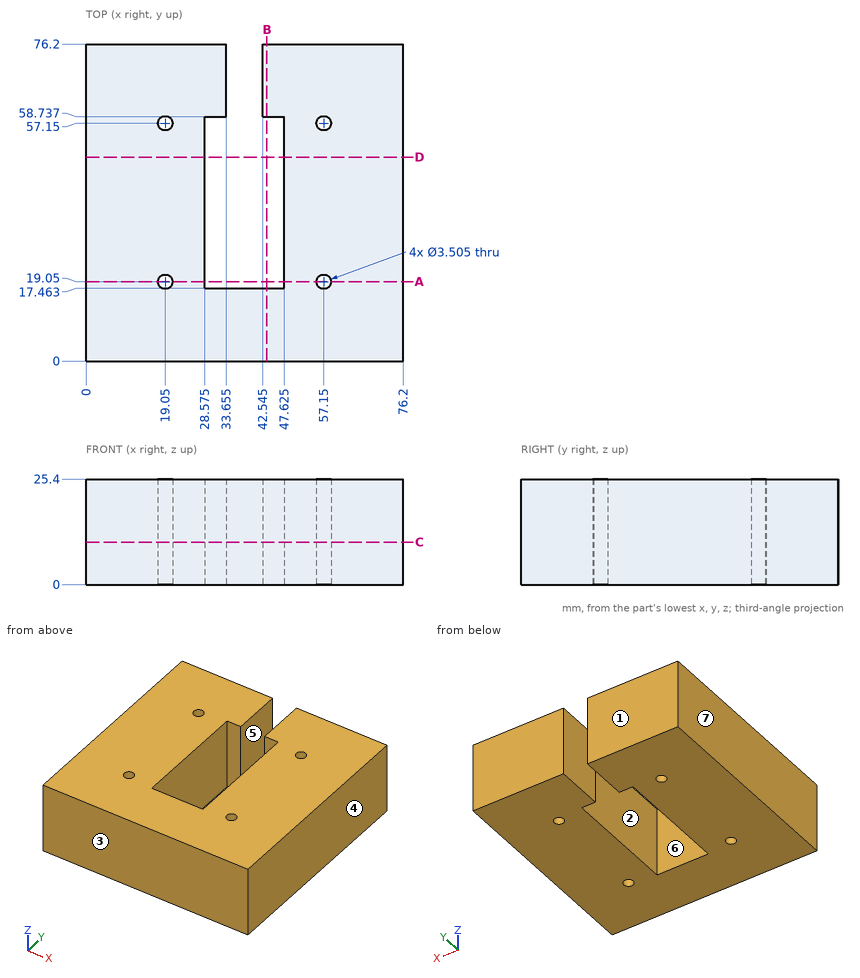
Geometry: see drawing. Coordinates: mm, zero at the bounding-box minimum. A direction names the side the tool comes from. Round coordinates to 2 decimals unless told otherwise and drop trailing zeros. Loops run counter-clockwise (first coordinate to the right, second up) from the corner with the lowest first, then second, coordinate; pieces in that order, holes last. Notation, with made-up numbers: (69, 37) - (85, 37) arc R21 ccw to (85, 50) - close; hole circle Ø6 at (73, 61.5). An arc over 180 degrees is marked (long way). Use CSV: the item, a comma, the result in double quotes.
Q1. Reachability of the marked faces 5, 6 and 7 from +Z, -Z, +X, -X, +Y, -Y: full face, straight path, thin tool, end or side. Return the list, or none.
Reported:
face 5,"+Z, -Z, +Y"
face 6,"+Z, -Z"
face 7,"+Z, -Z, -X, +Y, -Y"
Q2. Pin query (flat end, axial travel): pin 1 Ø3 at (x, y) = (57.15, 19.05) entering from +Z. Return the tip coordinate at first contact, or that it passes through.
Reported:
pin 1,"through"
Q3. Ray query, line 1 along Y through (x, z) = (19.05, 14); line 2 along X through (y, z) = (71.5, 22.5) (1 decimal); line 3 along Y through (x, z) = (46, 3.25). Return the intervals inside material, ascending.
Reported:
line 1,"0 to 17.3, 20.8 to 55.4, 58.9 to 76.2"
line 2,"0 to 33.7, 42.5 to 76.2"
line 3,"0 to 17.46, 58.74 to 76.2"
Q4. Section query A-A, the plane y = 19.05. Output: boundary loops of the cut face in (x, z) (1 decimal), then the cut area to 3 significant figures.
Reported:
outline,"(0, 0) - (17.3, 0) - (17.3, 25.4) - (0, 25.4) - close; (20.8, 0) - (28.6, 0) - (28.6, 25.4) - (20.8, 25.4) - close; (47.6, 0) - (55.4, 0) - (55.4, 25.4) - (47.6, 25.4) - close; (58.9, 0) - (76.2, 0) - (76.2, 25.4) - (58.9, 25.4) - close"
area,"1,270 mm^2"
Q5. Section query D-D, the plane y = 49. Output: boundary loops of the cut face in (x, z) (1 decimal), then the cut area to 3 significant figures.
Reported:
outline,"(0, 0) - (28.6, 0) - (28.6, 25.4) - (0, 25.4) - close; (47.6, 0) - (76.2, 0) - (76.2, 25.4) - (47.6, 25.4) - close"
area,"1,450 mm^2"
Q6. Section query B-B, the plane x = 43.5. Output: boundary loops of the cut face in (y, z).
Reported:
outline,"(0, 0) - (17.46, 0) - (17.46, 25.4) - (0, 25.4) - close; (58.74, 0) - (76.2, 0) - (76.2, 25.4) - (58.74, 25.4) - close"
Q7. Section query C-C, the plane z = 10.25. Give the number of separate pieces and of enclosed holes in the cut face, then the cut area to 3 significant figures.
Reported:
separate pieces,"1"
enclosed holes,"4"
area,"4,830 mm^2"
Q8. Mould query, pull axis Y, two halves, no side actions, for the marked faces 1, 2, 3 and 4. Classes: pulls with the +Y half, pulls with the -Y half, needs draft (parallel to the pull), parting line crosses it, or undercut.
Reported:
face 1,"pulls with the +Y half"
face 2,"undercut"
face 3,"pulls with the -Y half"
face 4,"needs draft"
